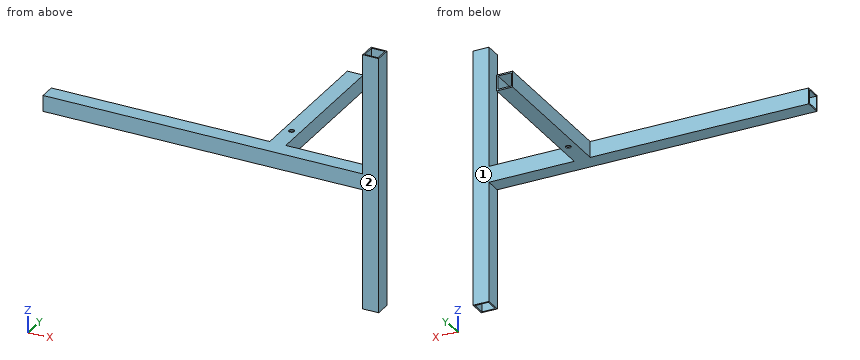
```python
from build123d import *

# Parameters (mm, degrees)
BOSS_EXTRUDE2_DEPTH      = 222.25
BOSS_EXTRUDE2_DEPTH_BACK = 539.75
SKETCH1_W                = 38.1
SKETCH1_H                = 38.1
SKETCH1_W_2              = 31.75
SKETCH1_H_2              = 31.75
SKETCH2_W                = 38.1
SKETCH2_H                = 38.1
SKETCH2_W_2              = 31.75
SKETCH2_H_2              = 31.75
BOSS_EXTRUDE3_DEPTH      = 355.6
SKETCH3_W                = 38.1
SKETCH3_H                = 38.1
SKETCH3_W_2              = 31.75
SKETCH3_H_2              = 31.75
BOSS_EXTRUDE4_DEPTH      = 304.8
SKETCH4_R                = 6.35
CUT_EXTRUDE1_DEPTH       = 743.434222676


with BuildPart() as part:
    # Sketch1 → Boss-Extrude2 (new, two sides: drawn at the far end of the back side and taken through both)
    with BuildSketch(Plane(origin=(0, 0, 0), x_dir=(0, 0, -1), z_dir=(1, 0, 0)).offset(-BOSS_EXTRUDE2_DEPTH_BACK)):
        with Locations((0, 19.05)):
            Rectangle(SKETCH1_W, SKETCH1_H)
        with Locations((0, 19.05)):
            Rectangle(SKETCH1_W_2, SKETCH1_H_2, mode=Mode.SUBTRACT)
    extrude(amount=BOSS_EXTRUDE2_DEPTH + BOSS_EXTRUDE2_DEPTH_BACK)

    # Sketch2 → Boss-Extrude3 (add)
    with BuildSketch(Plane(origin=(0, 38.1, 0), x_dir=(1, 0, 0), z_dir=(0, 1, 0))):
        Rectangle(SKETCH2_W, SKETCH2_H)
        Rectangle(SKETCH2_W_2, SKETCH2_H_2, mode=Mode.SUBTRACT)
    extrude(amount=BOSS_EXTRUDE3_DEPTH)

    # Sketch3 → Boss-Extrude4 (add, symmetric)
    with BuildSketch(Plane.XY):
        with Locations((241.3, 19.05)):
            Rectangle(SKETCH3_W, SKETCH3_H)
        with Locations((241.3, 19.05)):
            Rectangle(SKETCH3_W_2, SKETCH3_H_2, mode=Mode.SUBTRACT)
    extrude(amount=BOSS_EXTRUDE4_DEPTH, both=True)

    # Sketch4 → Cut-Extrude1 (cut, through all)
    with BuildSketch(Plane.XY.offset(19.05)):
        with Locations((0, 101.6)):
            Circle(SKETCH4_R)
    extrude(amount=-CUT_EXTRUDE1_DEPTH, mode=Mode.SUBTRACT)


solid = part.part
```
CAD build for the part. Positions are in the model's coordinates, mm. Face numbers are marked on the shaded views. A direction names the side the tool comes from. Coordinates: 2 decimals unless noted, no trailing zeros. Loops run counter-clockwise (first coordinate to the right, second up) from the corner with the lowest first, then second, coordinate; pieces in that order, holes last. Notation, with made-up numbers: (54.25, 45.25) - (67.25, 45.25) arc R9 ccw to (67.25, 52.25) - close; hole circle Ø5 at (-16.5, 59). An arc over 180 degrees is marked (long way). Use CSV: the item, a comma, the result in double quotes. Start each with the question number.
Q1. Drop flat-ended pins along their axis: P1, Ø11.5, axis at y = 152.5, z = -4, coming from the +X side; P2, Ø9.5, axis at x = -154.5, y = 23.5, coming from the +Z side; P3, Ø19, axis at y = 15, z = 179.5, coming from the -X side. Give the stop position or say it passes through.
Q2. Probe probe 1 along Y at (x, z) = (0, 17); probe 2 along Z at (x, y) = (8, 72) (3 decimals); probe 3 along Y at (x, z) = (-454, -16.5). List the from-to ranges inside material, lowest first. Write a range as from..to.
Q3. Cut at A-A, the plane y = 294.5. List the corners of the cut face in (x, z) (3 decimals).
Q4. Cut at B-B, the plane x = -145. List the corners of the cut face in (y, z) (3 decimals), then the cut area to 3 significant figures.
Q5. 3-axis set-ups, long thin cutter, end or side, ignore diameter. For the marked faces 1 and 2: which of +Z, -Z, +X, -X, +Y, -Y reach the whole face in a straight line?
Here are the results:
1,P1,"x = 19.05"
1,P2,"z = 19.05"
1,P3,"x = 222.25"
2,probe 1,"0..95.25, 107.95..393.7"
2,probe 2,"-19.05..-15.875, 15.875..19.05"
2,probe 3,"0..38.1"
3,outline,"(-19.05, -19.05) - (19.05, -19.05) - (19.05, 19.05) - (-19.05, 19.05) - close; hole (-15.875, -15.875) - (15.875, -15.875) - (15.875, 15.875) - (-15.875, 15.875) - close"
4,outline,"(0, -19.05) - (38.1, -19.05) - (38.1, 19.05) - (0, 19.05) - close; hole (3.175, -15.875) - (34.925, -15.875) - (34.925, 15.875) - (3.175, 15.875) - close"
4,area,"444 mm2"
5,face 1,"+Z, -Z, +X, +Y"
5,face 2,"+Z, -Z, +X, -X, -Y"
